Autodesk Inventor part; units mm, degrees
ref_plane "YZ Plane" through (0, 0, 0) normal (1, 0, 0) x (0, 1, 0)
ref_plane "XZ Plane" through (0, 0, 0) normal (0, 1, 0) x (-1, 0, 0)
ref_plane "XY Plane" through (0, 0, 0) normal (0, 0, 1) x (1, 0, 0)
sketch "Sketch3" plane through (0, 0, 0) normal (0, 0, 1) x (1, 0, 0)
  line L0 (0, 0) -> (812.8, 0) construction
  line L1 (812.8, 0) -> (812.8, -406.4) construction
  line L2 (812.8, -406.4) -> (0, -406.4) construction
  line L3 (0, -406.4) -> (0, 0) construction
  line L4 (406.4, 0) -> (0, 0)
  line L5 (0, -406.4) -> (0, 0)
  line L6 (0, -406.4) -> (406.4, -406.4)
  line L7 (406.4, 0) -> (406.4, -406.4)
  dimension "d88" = 812.8
extrude "Extrusion2" add sketch "Sketch3" against normal blind 406.4
sketch "Sketch4" plane through (0, 0, 0) normal (0, 0, 1) x (1, 0, 0)
  line L0 (0, 0) -> (406.4, 0)
  line L1 (0, 0) -> (812.8, 0) construction
  line L2 (812.8, 0) -> (812.8, -406.4) construction
  line L3 (812.8, -406.4) -> (0, -406.4) construction
  line L4 (0, -406.4) -> (0, 0) construction
  line L5 (0, 0) -> (25.4, 0)
  line L6 (25.4, 0) -> (25.4, -25.4)
  line L7 (25.4, -25.4) -> (0, -25.4)
  line L8 (0, -25.4) -> (0, 0)
  line L9 (25.4, -25.4) -> (381, -25.4)
  line L10 (381, -25.4) -> (381, -381)
  line L11 (381, -381) -> (25.4, -381)
  line L12 (25.4, -381) -> (25.4, -25.4)
  dimension "d95" = 812.8
  dimension "d102" = 25.4
  dimension "d103" = 25.4
  dimension "d104" = 355.6
  dimension "d105" = 355.6
extrude "Extrusion3" cut sketch "Sketch4" against normal blind 406.4 contours L9 L10 L11 L12
sketch "Sketch5" plane through (0, -406.4, 0) normal (-1, 0, 0) x (0, 0, 1)
  line L0 (0, 406.4) -> (-406.4, 406.4)
  line L1 (-406.4, 406.4) -> (-381, 406.4)
  line L2 (-381, 406.4) -> (-381, 381)
  line L3 (-381, 381) -> (-406.4, 381)
  line L4 (-406.4, 381) -> (-406.4, 406.4)
  line L5 (-381, 381) -> (-25.4, 381)
  line L6 (-25.4, 381) -> (-25.4, 25.4)
  line L7 (-25.4, 25.4) -> (-381, 25.4)
  line L8 (-381, 25.4) -> (-381, 381)
  dimension "d108" = 25.4
  dimension "d109" = 25.4
  dimension "d110" = 355.6
  dimension "d111" = 355.6
extrude "Extrusion4" cut sketch "Sketch5" against normal blind 406.4 contours L5 L6 L7 L8
sketch "Sketch6" plane through (0, 0, 0) normal (0, 1, 0) x (1, 0, 0)
  line L0 (0, 406.4) -> (406.4, 406.4)
  line L1 (0, 406.4) -> (25.4, 406.4)
  line L2 (25.4, 406.4) -> (25.4, 381)
  line L3 (25.4, 381) -> (0, 381)
  line L4 (0, 381) -> (0, 406.4)
  line L5 (25.4, 381) -> (381, 381)
  line L6 (381, 381) -> (381, 25.4)
  line L7 (381, 25.4) -> (25.4, 25.4)
  line L8 (25.4, 25.4) -> (25.4, 381)
  point P0 (0, 0)
  dimension "d114" = 25.4
  dimension "d115" = 25.4
  dimension "d116" = 355.6
  dimension "d117" = 355.6
extrude "Extrusion5" cut sketch "Sketch6" against normal blind 406.4 contours L5 L6 L7 L8
sketch "Sketch7" plane through (0, 0, 0) normal (0, 0, 1) x (1, 0, 0)
  point P0 (0, 0)
sketch "Sketch8" plane through (406.4, -381, -25.4) normal (0, 1, 0) x (1, 0, 0)
  line L0 (-381, 0) -> (-25.4, 0)
  line L1 (-25.4, 0) -> (-12.7, 0)
  line L2 (-25.4, 0) -> (0, 0)
  line L3 (0, 0) -> (-12.7, 0)
  line L4 (-25.4, 355.6) -> (0, 355.6)
  line L5 (-6.35, 0) -> (-19.05, 0)
  line L6 (-19.05, 0) -> (-19.05, 355.6)
  line L7 (-19.05, 355.6) -> (-6.35, 355.6)
  line L8 (-6.35, 355.6) -> (-6.35, 0)
  point P0 (-406.4, -25.4)
  point P1 (-19.05, 0)
  dimension "d120" = 12.7
extrude "Extrusion6" cut sketch "Sketch8" against normal blind 12.7
properties part number "JukeBox Metal Frame"
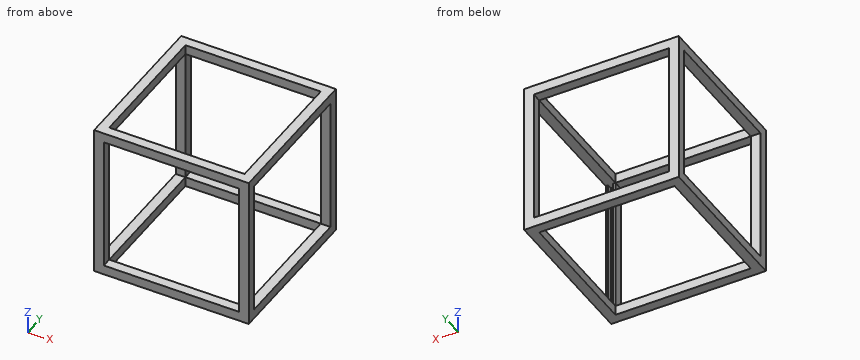
Source: CAD feature listing. Evaluate the final solid. Frame: model axes, mm. Give positions to 0.01 mm unless a question says otherwise; leave off trailing zeros. Loops run counter-clockwise (first coordinate to the right, second up) from the corner with the lowest first, then second, coordinate; pieces in that order, holes last. Notation, with made-up numbers: (32, 39) -> (51, 39) arc R18 cw to (51, 64) -> close; hole circle Ø8 at (54.5, 40). An arc over 180 degrees is marked (long way). Put each result on its own line as item: value. Start each with the question number.
1) Cut plane B-B (x = 263). Return loops of the section in (y, z), then the cut area to 3 significant figures.
2) Material intervals for probe 1 along X at (y, z) = (-33, -24); probe 2 along Y at (x, z) = (69, -381.5), sorted ascending.
3) Contact query for a flat-ended pin moving along its axis: P1, Ø14, axis at y = -385, z = -210, coming from the -X side. Output: stop coordinate, or through.
4) Cut plane A-A (z = -84.5). Return loops of the section in (x, y), then the cut area to 3 significant figures.
5) Cut plane C-C (y = -51.5). Return loops of the section in (x, z).
Results are:
1. outline: (-406.4, -406.4) -> (-381, -406.4) -> (-381, -381) -> (-406.4, -381) -> close; (-406.4, -25.4) -> (-381, -25.4) -> (-381, 0) -> (-406.4, 0) -> close; (-25.4, -406.4) -> (0, -406.4) -> (0, -381) -> (-25.4, -381) -> close; (-25.4, -25.4) -> (0, -25.4) -> (0, 0) -> (-25.4, 0) -> close
1. area: 2,580 mm2
2. probe 1: x = 0 to 25.4, 381 to 406.4
2. probe 2: y = -406.4 to -381, -25.4 to 0
3. P1: stops at x = 0
4. outline: (0, -406.4) -> (25.4, -406.4) -> (25.4, -381) -> (0, -381) -> close; (0, -25.4) -> (25.4, -25.4) -> (25.4, 0) -> (0, 0) -> close; (381, -406.4) -> (406.4, -406.4) -> (406.4, -381) -> (400.05, -381) -> (400.05, -393.7) -> (387.35, -393.7) -> (387.35, -381) -> (381, -381) -> close; (381, -25.4) -> (406.4, -25.4) -> (406.4, 0) -> (381, 0) -> close
4. area: 2,420 mm2
5. outline: (0, -406.4) -> (25.4, -406.4) -> (25.4, -381) -> (0, -381) -> close; (0, -25.4) -> (25.4, -25.4) -> (25.4, 0) -> (0, 0) -> close; (381, -406.4) -> (406.4, -406.4) -> (406.4, -381) -> (381, -381) -> close; (381, -25.4) -> (406.4, -25.4) -> (406.4, 0) -> (381, 0) -> close
